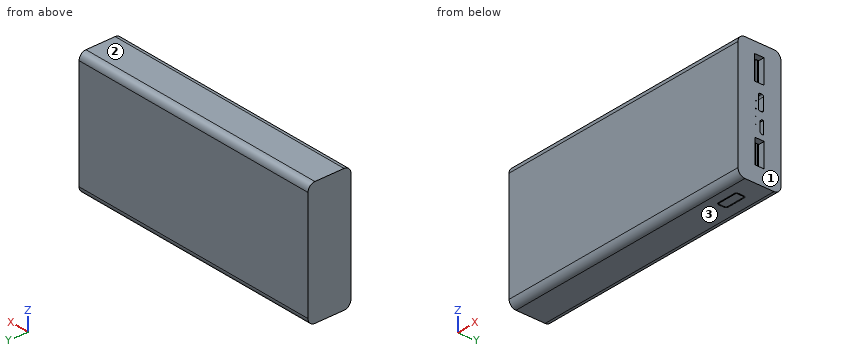
```python
from build123d import *

# Parameters (mm, degrees)
SKETCH_1_W          = 151
SKETCH_1_H          = 72
EXTRUDE_1_DEPTH     = 25
FILLET_1_R          = 4
FILLET_2_R          = 4
FILLET_3_R          = 4
FILLET_4_R          = 4
SKETCH_2_R          = 0.2
SKETCH_2_W          = 14
SKETCH_2_H          = 5.5
CUT_EXTRUDE_1_DEPTH = 15
SKETCH_3_W          = 12.373268072
SKETCH_3_H          = 1.582389444
SKETCH_3_W_2        = 7.077543374
SKETCH_3_H_2        = 0.5
SKETCH_3_W_3        = 3.808702178
SKETCH_3_H_3        = 0.2
EXTRUDE_2_DEPTH     = 13
CHAMFER_1_SIZE      = 0.5
CHAMFER_2_SIZE      = 0.5
CHAMFER_3_SIZE      = 0.5
CHAMFER_4_SIZE      = 0.5
CHAMFER_5_SIZE      = 0.5
CUT_EXTRUDE_2_DEPTH = 3


with BuildPart() as part:
    # 草图1 → 凸台-拉伸1 (new body)
    with BuildSketch(Plane(origin=(0, 0, 0), x_dir=(1, 0, 0), z_dir=(0, 1, 0))):
        with Locations((-21.814590862, -0.38165894)):
            Rectangle(SKETCH_1_W, SKETCH_1_H)
    extrude(amount=EXTRUDE_1_DEPTH)

    # 圆角1
    fillet_1_edges = [part.edges().sort_by_distance(p)[0] for p in [
        (-21.814590862, 25, 36.38165894),
    ]]
    fillet(fillet_1_edges, radius=FILLET_1_R)

    # 圆角2
    fillet_2_edges = [part.edges().sort_by_distance(p)[0] for p in [
        (-21.814590862, 25, -35.61834106),
    ]]
    fillet(fillet_2_edges, radius=FILLET_2_R)

    # 圆角3
    fillet_3_edges = [part.edges().sort_by_distance(p)[0] for p in [
        (-21.814590862, 0, 36.38165894),
    ]]
    fillet(fillet_3_edges, radius=FILLET_3_R)

    # 圆角4
    fillet_4_edges = [part.edges().sort_by_distance(p)[0] for p in [
        (-21.814590862, 0, -35.61834106),
    ]]
    fillet(fillet_4_edges, radius=FILLET_4_R)

    # 草图2 → 切除-拉伸1 (cut)
    with BuildSketch(Plane(origin=(53.685409138, 0, 0), x_dir=(0, 0, -1), z_dir=(1, 0, 0))):
        with Locations((-6.38165894, 10.438981293)):
            Circle(SKETCH_2_R)
        with Locations((-2.38165894, 10.438981293)):
            Circle(SKETCH_2_R)
        with Locations((1.61834106, 10.438981293)):
            Circle(SKETCH_2_R)
        with Locations((5.61834106, 10.438981293)):
            Circle(SKETCH_2_R)
        with Locations((-23.032936311, 12.408130846)):
            Rectangle(SKETCH_2_W, SKETCH_2_H)
        with BuildLine():
            Line((-10.032936311, 14.854810604), (-3.032936311, 14.854810604))
            ThreePointArc((-3.032936311, 14.854810604), (-2.32582953, 14.561917385), (-2.032936311, 13.854810604))
            Line((-2.032936311, 13.854810604), (-2.032936311, 12.854810604))
            ThreePointArc((-2.032936311, 12.854810604), (-2.32582953, 12.147703823), (-3.032936311, 11.854810604))
            Line((-3.032936311, 11.854810604), (-10.032936311, 11.854810604))
            ThreePointArc((-10.032936311, 11.854810604), (-10.740043093, 12.147703823), (-11.032936311, 12.854810604))
            Line((-11.032936311, 12.854810604), (-11.032936311, 13.854810604))
            ThreePointArc((-11.032936311, 13.854810604), (-10.740043093, 14.561917385), (-10.032936311, 14.854810604))
        make_face()
        Polygon((1.967063689, 14.74117963), (9.467063689, 14.74117963), (9.467063689, 13.74117963), (8.467063689, 12.74117963), (2.967063689, 12.74117963), (1.967063689, 13.74117963), align=None)
        with Locations((19.400712994, 12.527228442)):
            Rectangle(SKETCH_2_W, SKETCH_2_H)
    extrude(amount=-CUT_EXTRUDE_1_DEPTH, mode=Mode.SUBTRACT)

    # 草图3 → 凸台-拉伸2 (add)
    with BuildSketch(Plane(origin=(38.685409138, 0, 0), x_dir=(0, 0, -1), z_dir=(1, 0, 0))):
        with Locations((-23.032936311, 13.344739888)):
            Rectangle(SKETCH_3_W, SKETCH_3_H)
        with Locations((19.400712994, 13.344739888)):
            Rectangle(SKETCH_3_W, SKETCH_3_H)
        with Locations((-6.532936311, 13.198610031)):
            Rectangle(SKETCH_3_W_2, SKETCH_3_H_2)
        with Locations((5.717063689, 13.913029352)):
            Rectangle(SKETCH_3_W_3, SKETCH_3_H_3)
    extrude(amount=EXTRUDE_2_DEPTH)

    # 倒角1
    chamfer_1_edges = [part.edges().sort_by_distance(p)[0] for p in [
        (51.685409138, 12.553545166, 23.032936311),
    ]]
    chamfer(chamfer_1_edges, length=CHAMFER_1_SIZE)

    # 倒角2
    chamfer_2_edges = [part.edges().sort_by_distance(p)[0] for p in [
        (51.685409138, 14.13593461, 23.032936311),
    ]]
    chamfer(chamfer_2_edges, length=CHAMFER_2_SIZE)

    # 倒角3
    chamfer_3_edges = [part.edges().sort_by_distance(p)[0] for p in [
        (51.685409138, 13.344739888, 29.219570347),
    ]]
    chamfer(chamfer_3_edges, length=CHAMFER_3_SIZE)

    # 倒角4
    chamfer_4_edges = [part.edges().sort_by_distance(p)[0] for p in [
        (51.685409138, 13.344739888, 16.846302275),
    ]]
    chamfer(chamfer_4_edges, length=CHAMFER_4_SIZE)

    # 倒角5
    chamfer_5_edges = [part.edges().sort_by_distance(p)[0] for p in [
        (51.685409138, 13.344739888, -13.214078958),
        (51.685409138, 12.553545166, -19.400712994),
        (51.685409138, 13.344739888, -25.58734703),
        (51.685409138, 14.13593461, -19.400712994),
    ]]
    chamfer(chamfer_5_edges, length=CHAMFER_5_SIZE)

    # 草图4 → 切除-拉伸2 (cut)
    with BuildSketch(Plane(origin=(0, 0, -35.61834106), x_dir=(-1, 0, 0), z_dir=(0, 0, -1))):
        with BuildLine():
            Line((-40.885409138, 14.323868956), (-30.485409138, 14.323868956))
            ThreePointArc((-30.485409138, 14.323868956), (-29.884368374, 14.07490972), (-29.635409138, 13.473868956))
            Line((-29.635409138, 13.473868956), (-29.635409138, 10.378810207))
            ThreePointArc((-29.635409138, 10.378810207), (-29.884368374, 9.777769443), (-30.485409138, 9.528810207))
            Line((-30.485409138, 9.528810207), (-40.885409138, 9.528810207))
            ThreePointArc((-40.885409138, 9.528810207), (-41.486449902, 9.777769443), (-41.735409138, 10.378810207))
            Line((-41.735409138, 10.378810207), (-41.735409138, 13.473868956))
            ThreePointArc((-41.735409138, 13.473868956), (-41.486449902, 14.07490972), (-40.885409138, 14.323868956))
        make_face()
        with BuildLine():
            Line((-40.885409138, 14.273868956), (-30.485409138, 14.273868956))
            ThreePointArc((-30.485409138, 14.273868956), (-29.919723713, 14.03955438), (-29.685409138, 13.473868956))
            Line((-29.685409138, 13.473868956), (-29.685409138, 10.378810207))
            ThreePointArc((-29.685409138, 10.378810207), (-29.919723713, 9.813124782), (-30.485409138, 9.578810207))
            Line((-30.485409138, 9.578810207), (-40.885409138, 9.578810207))
            ThreePointArc((-40.885409138, 9.578810207), (-41.451094563, 9.813124782), (-41.685409138, 10.378810207))
            Line((-41.685409138, 10.378810207), (-41.685409138, 13.473868956))
            ThreePointArc((-41.685409138, 13.473868956), (-41.451094563, 14.03955438), (-40.885409138, 14.273868956))
        make_face(mode=Mode.SUBTRACT)
    extrude(amount=-CUT_EXTRUDE_2_DEPTH, mode=Mode.SUBTRACT)

    # 切除-扫描1: sweep along a path in 草图5
    with BuildLine(Plane(origin=(0, 0, -35.61834106), x_dir=(-1, 0, 0), z_dir=(0, 0, -1))) as sweep_1_path:
        Line((-40.935409138, 14.823868956), (-30.435409138, 14.823868956))
        ThreePointArc((-30.435409138, 14.823868956), (-29.516170322, 14.443107771), (-29.135409138, 13.523868956))
        Line((-29.135409138, 13.523868956), (-29.135409138, 10.328810207))
        ThreePointArc((-29.135409138, 10.328810207), (-29.516170322, 9.409571391), (-30.435409138, 9.028810207))
        Line((-30.435409138, 9.028810207), (-40.935409138, 9.028810207))
        ThreePointArc((-40.935409138, 9.028810207), (-41.854647953, 9.409571391), (-42.235409138, 10.328810207))
        Line((-42.235409138, 10.328810207), (-42.235409138, 13.523868956))
        ThreePointArc((-42.235409138, 13.523868956), (-41.854647953, 14.443107771), (-40.935409138, 14.823868956))
    # 草图6 → 切除-扫描1 (sweep, cut)
    with BuildSketch(Plane(origin=(0, 11, 0), x_dir=(1, 0, 0), z_dir=(0, 1, 0))):
        with BuildLine():
            Line((41.735409138, 35.51679266), (41.735409138, 35.61834106))
            Line((41.735409138, 35.61834106), (42.235409138, 35.61834106))
            add(Edge.make_bspline(
                [(42.235409138, 35.61834106), (42.184892706, 35.515744093), (41.735409138, 35.51679266)],
                knots=[0, 0, 0, 1, 1, 1], degree=2))
        make_face()
    sweep(path=sweep_1_path.line, mode=Mode.SUBTRACT)


solid = part.part
```
CAD build for the part. Positions are in the model's coordinates, mm. Face numbers are marked on the shaded views. Give positions to 0.01 mm unless a question says otherwise; leave off trailing zeros. Order: outer loops, then holes, each group sorted by start corner. A loop starts at its lowest first (then second) coordinate and runs counter-clockwise, first axis right, second up. Notation, with made-up numbers: M 28,75 L 75,75 A17 cw 75,81 Z; hole C 35,9.5 d1. An arc over 180 degrees is marked long. Put each result on its own line as item: value. Start each with the question number.
(1) Mould opens along Z. For the marked faces 1, 2 and 3 say: +Z half, -Z half, draft (parallel to the pull), parting line (faces both ways), or undercut.
(2) Drill centre lines: line 1 along X through (y, z) = (12.25, 24.5); line 2 along Z through (x, y) = (18.5, 21.5); line 3 along Z through (x, y) = (0, 2.5). Where is each one in solid material? Low to high.
(3) Saw through at A-A, the plane z = -15.5. Write the cut outline in (x, y).
(4) Flat gauge pins, fed straight in: pin 1 Ø0.9 at (x, z) = (36, -33.5) entering from +Y (3 decimals); pin 2 Ø6 at (y, z) = (12, 23) entering from +X; pin 3 Ø1 at (y, z) = (13.5, -5.5) entering from +X. Where does each tip first touch, or does it go through?
Check result:
1. face 1: draft
1. face 2: +Z half
1. face 3: -Z half
2. line 1: x = -97.31 to 38.69
2. line 2: z = -35.59 to 36.35
2. line 3: z = -35.33 to 36.09
3. outline: M -97.31,0 L 53.69,0 L 53.69,9.78 L 38.69,9.78 L 38.69,12.55 L 51.19,12.55 L 51.69,13.05 L 51.69,13.64 L 51.19,14.14 L 38.69,14.14 L 38.69,15.28 L 53.69,15.28 L 53.69,25 L -97.31,25 Z
4. pin 1: stops at y = 24.735
4. pin 2: stops at x = 53.69
4. pin 3: stops at x = 51.69
